CAD build for the part. Positions are in the model's coordinates, mm. A direction names the side the tool comes from. Round coordinates to 2 decimals unless told otherwise and drop trailing zeros. Write each loop counter-clockwise with the first axis right and the second up, starting at its lowest first coordinate (ties: lowest second). Pieces come first, ordered by that corner, then holes. Notation, with made-up numbers: (-19, -15.5) -> (29, -15.5) arc R15 cw to (29, 6.5) -> close; hole circle Ø6 at (4.5, 89). An arc over 180 degrees is marked (long way). Put each result on its own line as item: value. Start each with the question number.
1. Saw through at C-C on y = 18. List the corners of the cut face in (x, z).
2. Saw through at B-B on z = -12.7. List the corners of the cut face in (x, y), and give its area (3 significant figures).
3. Flat gauge pins, fed straight in: P1, Ø2, axis at y = 21, z = -11.5, coming from the +X side; P2, Ø2.5, axis at x = 12.5, z = 13.5, coming from the -Y side; P3, Ø3.5, axis at x = -25, y = 8, coming from the -Z side. Where does each tip first touch, or does it go through?
4. Pull direction Z, two halves, no side cores. Call faces 1 (the flat face through (0, 35, 0)), 2 (the cylindrical face through (12.37, 32.53, 10.22)), 3 (the flat face through (-4, 0, -23)): pulls with the +Z half, pulls with the -Z half, needs draft (parallel to the pull), parting line crosses it, or undercut.
5. Drill centre lines: line 1 (X direction, y = 16.5, z = 0.5); line 2 (Z direction, x = 12.7, y = 31.1); line 3 (Z direction, x = 0, y = 8.5). Where is each one in solid material? Low to high. Write a range as from..to.
6. Saw through at A-A on y = 32. State how many separate pieces and enclosed holes the cut face has, and give its area (3 significant figures).
7. 3-axis set-ups, long thin cutter, end or side, ignore diameter. For faces 4 (the flat face through (0, 40, 0)), 5 (the cylindrical face through (-21.938, 17.255, -6.909)), 6 (the flat face through (24, 6, 2.25)): which of +Z, -Z, +X, -X, +Y, -Y reach the whole face in a straight line?
Autodesk Inventor part; units mm, degrees
ref_plane "XZ Plane" through (0, 0, 0) normal (0, 1, 0) x (-1, 0, 0)
ref_plane "XY Plane" through (0, 0, 0) normal (0, 0, 1) x (1, 0, 0)
sketch "Sketch1" plane through (0, 0, 0) normal (0, 1, 0) x (-1, 0, 0)
  circle A0 centre (0, 0) radius 23
  circle A1 centre (0, 0) radius 26
  dimension "d0" = 46
  dimension "d1" = 52
extrude "Extrusion1" add sketch "Sketch1" along normal blind 35
sketch "Sketch2" plane through (0, 35, 0) normal (0, 1, 0) x (1, 0, 0)
  circle A0 centre (0, 0) radius 26
extrude "Extrusion2" add sketch "Sketch2" along normal blind 5
sketch "Sketch3" plane through (0, 35, 0) normal (0, -1, 0) x (1, 0, 0)
  line L0 (-12.7, 12.7) -> (12.7, 12.7)
  line L1 (12.7, 12.7) -> (12.7, -12.7)
  line L2 (12.7, -12.7) -> (-12.7, -12.7)
  line L3 (-12.7, -12.7) -> (-12.7, 12.7)
  line L4 (-12.7, 12.7) -> (12.7, -12.7) construction
  line L5 (12.7, 12.7) -> (-12.7, -12.7) construction
  circle A0 centre (12.7, 12.7) radius 2.5
  circle A1 centre (12.7, -12.7) radius 2.5
  circle A2 centre (-12.7, -12.7) radius 2.5
  circle A3 centre (-12.7, 12.7) radius 2.5
  circle A4 centre (12.7, 12.7) radius 1
  circle A5 centre (12.7, -12.7) radius 1
  circle A6 centre (-12.7, -12.7) radius 1
  circle A7 centre (-12.7, 12.7) radius 1
  point P0 (0, 0)
  dimension "d6" = 25.4
  dimension "d7" = 25.4
  dimension "d8" = 5
  dimension "d9" = 5
  dimension "d10" = 5
  dimension "d11" = 5
  dimension "d14" = 2
  dimension "d15" = 2
  dimension "d16" = 2
  dimension "d17" = 2
extrude "Extrusion3" add sketch "Sketch3" along normal blind 5 contours A7 L3 A3 L0 | L0 A3 L3 A7 | A0 L1 A4 L0 | L0 A4 L1 A0 | A2 L2 A6 L3 | L3 A6 L2 A2 | A1 L2 A5 L1 | L1 A5 L2 A1
ref_plane "Work Plane1" through (26, 0, 0) normal (1, 0, 0) x (0, 1, 0)
sketch "Sketch4" plane through (26, 0, 0) normal (1, 0, 0) x (0, 1, 0)
  line L0 (0, 0) -> (12.5, 0) construction
  line L1 (0, -2.25) -> (12.5, -2.25)
  line L2 (12.5, 2.25) -> (0, 2.25)
  arc A0 (0, 2.25) -> (0, -2.25) centre (0, 0) ccw
  arc A1 (12.5, -2.25) -> (12.5, 2.25) centre (12.5, 0) ccw
  point P0 (0, 0)
  point P1 (6.25, 0)
  dimension "d19" = 12.5
  dimension "d20" = 4.5
extrude "Extrusion4" cut sketch "Sketch4" against normal through all
properties part number "TopPotentiometer_3DPrint"
Return value:
1. outline: circle Ø52 at (0, 0); hole circle Ø46 at (0, 0)
2. outline: (-22.69, 0) -> (-19.18, 0) -> (-19.18, 35) -> (-15.2, 35) -> (-15.2, 30) -> (-13.7, 30) -> (-13.7, 35) -> (-11.7, 35) -> (-11.7, 30) -> (-10.2, 30) -> (-10.2, 35) -> (10.2, 35) -> (10.2, 30) -> (11.7, 30) -> (11.7, 35) -> (13.7, 35) -> (13.7, 30) -> (15.2, 30) -> (15.2, 35) -> (19.18, 35) -> (19.18, 0) -> (22.69, 0) -> (22.69, 40) -> (-22.69, 40) -> close
2. area: 503 mm^2
3. P1: stops at x = 23.79
3. P2: stops at y = 30
3. P3: stops at z = -11.64
4. face 1: undercut
4. face 2: undercut
4. face 3: needs draft
5. line 1: x = -26..-22.99, 22.99..26
5. line 2: z = -22.69..-19.18, -15.2..-13.7, -11.7..-10.2, 10.2..11.7, 13.7..15.2, 19.18..22.69
5. line 3: z = -26..-23, 23..26
6. separate pieces: 5
6. enclosed holes: 5
6. area: 528 mm^2
7. face 4: +Z, -Z, +X, -X, +Y
7. face 5: -Y
7. face 6: +X, -X, -Y
